```python
from build123d import *

# Parameters (mm, degrees)
CROQUIS1_W              = 3
CROQUIS1_H              = 47
SALIENTE_EXTRUIR1_DEPTH = 3
CROQUIS2_W              = 3
CROQUIS2_H              = 1
SALIENTE_EXTRUIR2_DEPTH = 20
CROQUIS3_W              = 3
CROQUIS3_H              = 4
SALIENTE_EXTRUIR3_DEPTH = 11.48
CROQUIS4_W              = 3
CROQUIS4_H              = 3
SALIENTE_EXTRUIR4_DEPTH = 10
SALIENTE_EXTRUIR5_DEPTH = 5


with BuildPart() as part:
    # Croquis1 → Saliente-Extruir1 (new body)
    with BuildSketch(Plane.XY):
        with Locations((1.5, 23.5)):
            Rectangle(CROQUIS1_W, CROQUIS1_H)
    extrude(amount=SALIENTE_EXTRUIR1_DEPTH)

    # Croquis2 → Saliente-Extruir2 (add)
    with BuildSketch(Plane(origin=(0, 47, 0), x_dir=(1, 0, 0), z_dir=(0, 1, 0))):
        with Locations((1.5, -2.5)):
            Rectangle(CROQUIS2_W, CROQUIS2_H)
    extrude(amount=SALIENTE_EXTRUIR2_DEPTH)

    # Croquis3 → Saliente-Extruir3 (add)
    with BuildSketch(Plane.XY.offset(3)):
        with Locations((1.5, 2)):
            Rectangle(CROQUIS3_W, CROQUIS3_H)
    extrude(amount=SALIENTE_EXTRUIR3_DEPTH)

    # Croquis4 → Saliente-Extruir4 (add)
    with BuildSketch(Plane(origin=(0, 4, 0), x_dir=(1, 0, 0), z_dir=(0, 1, 0))):
        with Locations((1.5, -15.98)):
            Rectangle(CROQUIS4_W, CROQUIS4_H)
    extrude(amount=-SALIENTE_EXTRUIR4_DEPTH)

    # Croquis5 → Saliente-Extruir5 (add)
    with BuildSketch(Plane.ZY):
        Polygon((14.48, 0), (3, 0), (3, 4), (17.48, 4), (17.48, -6), (14.48, -6), align=None)
    extrude(amount=SALIENTE_EXTRUIR5_DEPTH)


solid = part.part
```
Check sheet for the modelled part. Datum: model origin and axes. Units: mm. A direction names the side the tool comes from. Round coordinates to 2 decimals unless told otherwise and drop trailing zeros. Order: outer loops, then holes, each group sorted by start corner. A loop starts at its lowest first (then second) coordinate and runs counter-clockwise, first axis right, second up. Notation, with made-up numbers: M 19,-7.5 L 51,-7.5 A24 ccw 51,21.5 Z; hole C -13.5,-40 d2. An arc over 180 degrees is marked long. Answer in a Markdown table with one row per item.
(1) Section check A-A on x = 1.75. Record the boundary of the cut face in (y, z).
Findings:
| item | result |
|---|---|
| outline | M -6,14.48 L 0,14.48 L 0,0 L 47,0 L 47,2 L 67,2 L 67,3 L 4,3 L 4,17.48 L -6,17.48 Z |
(2) Draft check along X on faces 6 (the flat face through (-1, -3, 14.48)), 7 (the flat face through (3, 20, 2)), 8 (the flat face through (0, 27, 2)). Enter one of: +X half, -X half, draft (parallel to the pull), parting line (faces both ways), or undercut.
Findings:
| item | result |
|---|---|
| face 6 | draft |
| face 7 | +X half |
| face 8 | -X half |
(3) Section check B-B on y = 38. Record the boundary of the cut face in (x, z), plus the area to 3 significant figures.
Findings:
| item | result |
|---|---|
| outline | M 0,0 L 3,0 L 3,3 L 0,3 Z |
| area | 9.00 mm^2 |
(4) Material ranges on line 1 along Y through (x, z) = (2.75, 9); line 2 along Z through (x, y) = (0.5, 13); line 3 along Z through (x, y) = (1.75, 60), recorded low to high. Write a range as from..to.
Findings:
| item | result |
|---|---|
| line 1 | y = 0..4 |
| line 2 | z = 0..3 |
| line 3 | z = 2..3 |
(5) Section check D-D on x = -3.25. Record the boundary of the cut face in (y, z).
Findings:
| item | result |
|---|---|
| outline | M -6,14.48 L 0,14.48 L 0,3 L 4,3 L 4,17.48 L -6,17.48 Z |
(6) Gauge pin test, flat ends, axial feed: pin 1 (4 mm diameter, centred on x = 1.5, y = 56.5, fed in from +Z); pin 2 (4 mm diameter, centred on x = -4, z = 8.5, fed in from +Y); pin 3 (2.5 mm diameter, centred on y = 22, z = 1, fed in from -X). Record the tip position at first contact, or that the pin passes through.
Findings:
| item | result |
|---|---|
| pin 1 | stops at z = 3 |
| pin 2 | stops at y = 4 |
| pin 3 | stops at x = 0 |
(7) Set-up check for faces 1 (the flat face through (-2, 2, 3)), 2 (the flat face through (-1, -6, 16)), 3 (the flat face through (-1, 4, 10)), 4 (the flat face through (1, 47, 1)), 5 (the flat face through (-1, 0, 9)): record each of +Z, -Z, +X, -X, +Y, -Y from which the full face is reachable in a straight line by a thin tool's end or side.
Findings:
| item | result |
|---|---|
| face 1 | -Z, -X, +Y, -Y |
| face 2 | +Z, -Z, +X, -X, -Y |
| face 3 | +Z, +X, -X, +Y |
| face 4 | -Z, +X, -X, +Y |
| face 5 | -Z, +X, -X, -Y |
(8) Section check C-C on z = 9.25. Record the boundary of the cut face in (x, y).
Findings:
| item | result |
|---|---|
| outline | M -5,0 L 3,0 L 3,4 L -5,4 Z |
